Part print with two shaded views. Sizes in mm from the minimum x, y, z corner. A direction names the side the tool comes from. Round coordinates to 2 decimals unless told otherwise and drop trailing zeros. Loops run counter-clockwise (first coordinate to the right, second up) from the corner with the lowest first, then second, coordinate; pieces in that order, holes last. Notation, with made-up numbers: (-7.5, 53.25) -> (-0.5, 53.25) arc R18 ccw to (-0.5, 64.25) -> close; hole circle Ø10 at (-6.5, -1). An arc over 180 degrees is marked (long way). Use a Markdown table: item, result. Add a question column.
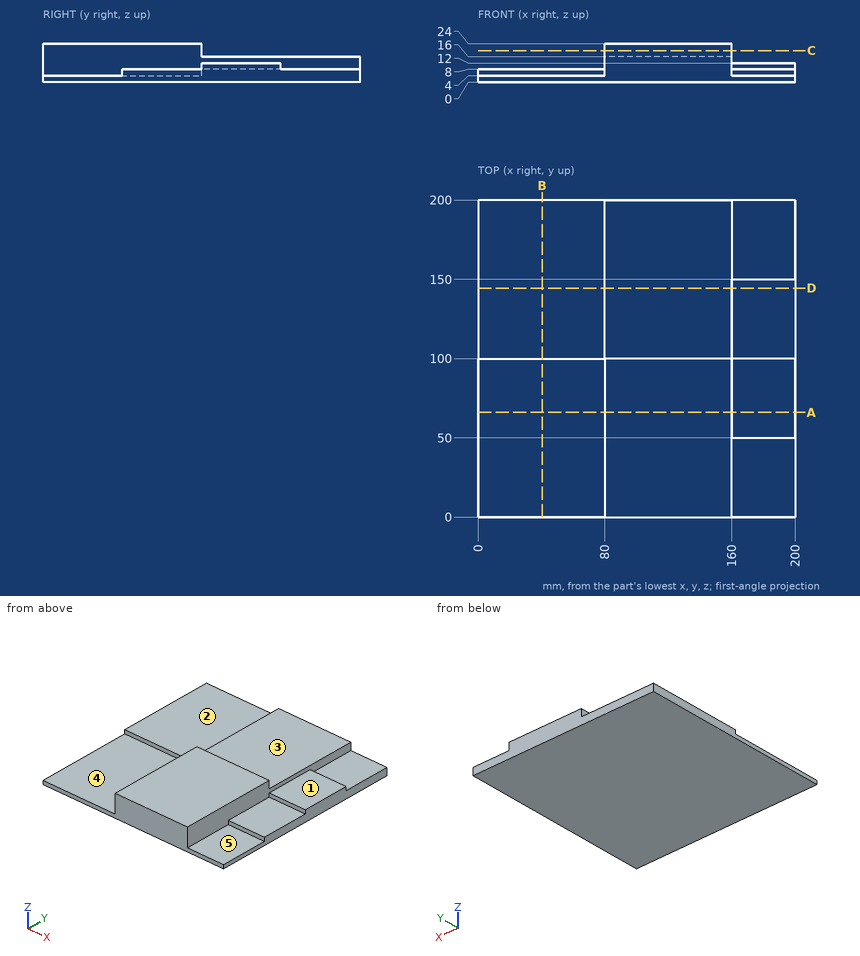
1) Cut at C-C on z = 19.75. Write the cut outline in (x, y), and give its area (3 significant figures).
2) Cut at A-A on y = 66. Write the cut outline in (x, z), and give its area (3 significant figures).
3) Pin check, flat tips, straight feed: pin 1 Ø2 at (x, z) = (171, 10.5) entering from +Y; pin 2 Ø2 at (x, z) = (53.5, 6) entering from -Y; pin 3 Ø2.5 at (x, z) = (138, 20.5) entering from +Y; pin 4 Ø4 at (x, z) = (98.5, 13.5) entering from -Y. Stop position of each tip, or through.
4) Cut at D-D on y = 144.5. Write the cut outline in (x, z).
5) Cut at B-B on x = 40.5. Write the cut outline in (y, z), and give its area (3 significant figures).
6) Tool access for the marked faces 1, 2, 3, 4 and 5: list every direction of +Z, -Z, +X, -X, +Y, -Y with a clear straight run to the whole face (end or side of a thin tool).
7) Wall check: probe 1 along Y at (x, z) = (109.5, 19); probe 2 along X at (y, z) = (83.5, 19.5); probe 3 along Z at (x, y) = (160.5, 62). Give the ranges that are in metal, low to high. Write a range as from..to.
Established:
| question | item | result |
|---|---|---|
| 1 | outline | (80, 0) -> (160, 0) -> (160, 100) -> (80, 100) -> close |
| 1 | area | 8,000 mm^2 |
| 2 | outline | (0, 0) -> (200, 0) -> (200, 8) -> (160, 8) -> (160, 24) -> (80, 24) -> (80, 4) -> (0, 4) -> close |
| 2 | area | 2,560 mm^2 |
| 3 | pin 1 | stops at y = 150 |
| 3 | pin 2 | stops at y = 100 |
| 3 | pin 3 | stops at y = 100 |
| 3 | pin 4 | stops at y = 0 |
| 4 | outline | (0, 0) -> (200, 0) -> (200, 12) -> (160, 12) -> (160, 16) -> (80, 16) -> (80, 8) -> (0, 8) -> close |
| 5 | outline | (0, 0) -> (200, 0) -> (200, 8) -> (100, 8) -> (100, 4) -> (0, 4) -> close |
| 5 | area | 1,200 mm^2 |
| 6 | face 1 | +Z, +X, +Y, -Y |
| 6 | face 2 | +Z, -X, +Y, -Y |
| 6 | face 3 | +Z, +X, -X, +Y |
| 6 | face 4 | +Z, -X, -Y |
| 6 | face 5 | +Z, +X, -Y |
| 7 | probe 1 | y = 0..100 |
| 7 | probe 2 | x = 80..160 |
| 7 | probe 3 | z = 0..8 |
